The drawing under review shows one solid part. Ordinate dimensions are in mm from its lowest x, y, z. A direction names the side the tool comes from. Give positions to 0.01 mm unless a question says otherwise; leave off trailing zeros. Write each loop counter-clockwise with the first axis right and the second up, starting at its lowest first coordinate (ties: lowest second). Pieces come first, ordered by that corner, then holes. Notation, with made-up numbers: (-4, 87.5) -> (32, 87.5) arc R15 ccw to (32, 114.5) -> close; hole circle Ø6 at (-1.5, 50). An arc over 180 degrees is marked (long way). Put each result on its own line as item: value. Start each with the question number.
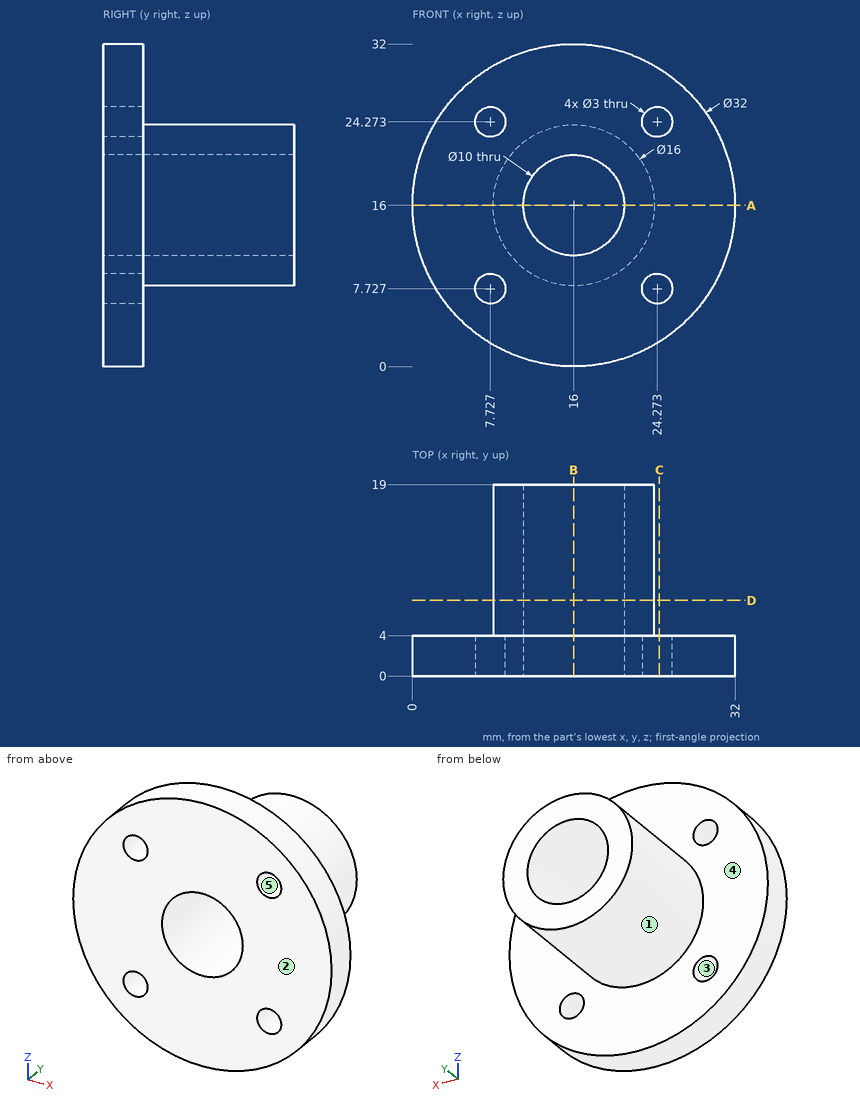
Q1. Take a section at B-B on x = 16. Give the boundary of the cut face in (y, z).
Q2. To check wall thickness, follow probe 1 along X at (y, z) = (7.5, 16); probe 2 along Y at (x, z) = (6.5, 19.5); probe 3 along Z at (x, y) = (15, 7). State the ranges of each line that lie inside material, in increasing order. Write a range as from..to.
Q3. Take a section at C-C on x = 24.5. Give the boundary of the cut face in (y, z), then the cut area to 3 significant figures.
Q4. For pin 1 (3 mm diameter, centred on x = 13.5, y = 11, fed in from +Z); pin 2 (3 mm diameter, centred on x = 20, y = 15.5, fed in from -Z); pin 3 (5 mm diameter, centred on x = 7.73, z = 24.27, fed in from +Y); pin 4 (2.5 mm diameter, centred on x = 24.27, z = 7.73, fed in from +Y), all flat-tipped, find the tip position at first contact; note any pin that passes through.
Q5. Take a section at D-D on y = 7.5. Give the boundary of the cut face in (x, z), then the cut area to 4 significant figures.
Q6. Take a section at A-A on z = 16. Give the boundary of the cut face in (x, y).
Q7. Mouldability with a two-part tool opening along X and no side actions: class the marked faces 1, 2 and 3 as +X half, -X half, draft (parallel to the pull), parting line (faces both ways), or undercut.
Q8. Machinability: for the marked faces 4 and 5, which of the approach directions +Z, -Z, +X, -X, +Y, -Y give a long, thin tool a straight path to every point of the face, cutting with its end or side? Answer none if there is none.
Result:
1. outline: (0, 0) -> (4, 0) -> (4, 8) -> (19, 8) -> (19, 11) -> (0, 11) -> close; (0, 21) -> (19, 21) -> (19, 24) -> (4, 24) -> (4, 32) -> (0, 32) -> close
2. probe 1: x = 8..11, 21..24
2. probe 2: y = 0..4
2. probe 3: z = 8.06..11.1, 20.9..23.94
3. outline: (0, 2.44) -> (4, 2.44) -> (4, 6.24) -> (0, 6.24) -> close; (0, 9.21) -> (4, 9.21) -> (4, 22.79) -> (0, 22.79) -> close; (0, 25.76) -> (4, 25.76) -> (4, 29.56) -> (0, 29.56) -> close
3. area: 84.7 mm^2
4. pin 1: stops at z = 23.94
4. pin 2: stops at z = 8.4
4. pin 3: stops at y = 4
4. pin 4: passes through
5. outline: circle Ø16 at (16, 16); hole circle Ø10 at (16, 16)
5. area: 122.5 mm^2
6. outline: (0, 0) -> (11, 0) -> (11, 19) -> (8, 19) -> (8, 4) -> (0, 4) -> close; (21, 0) -> (32, 0) -> (32, 4) -> (24, 4) -> (24, 19) -> (21, 19) -> close
7. face 1: parting line
7. face 2: draft
7. face 3: undercut
8. face 4: +Y
8. face 5: +Y, -Y
